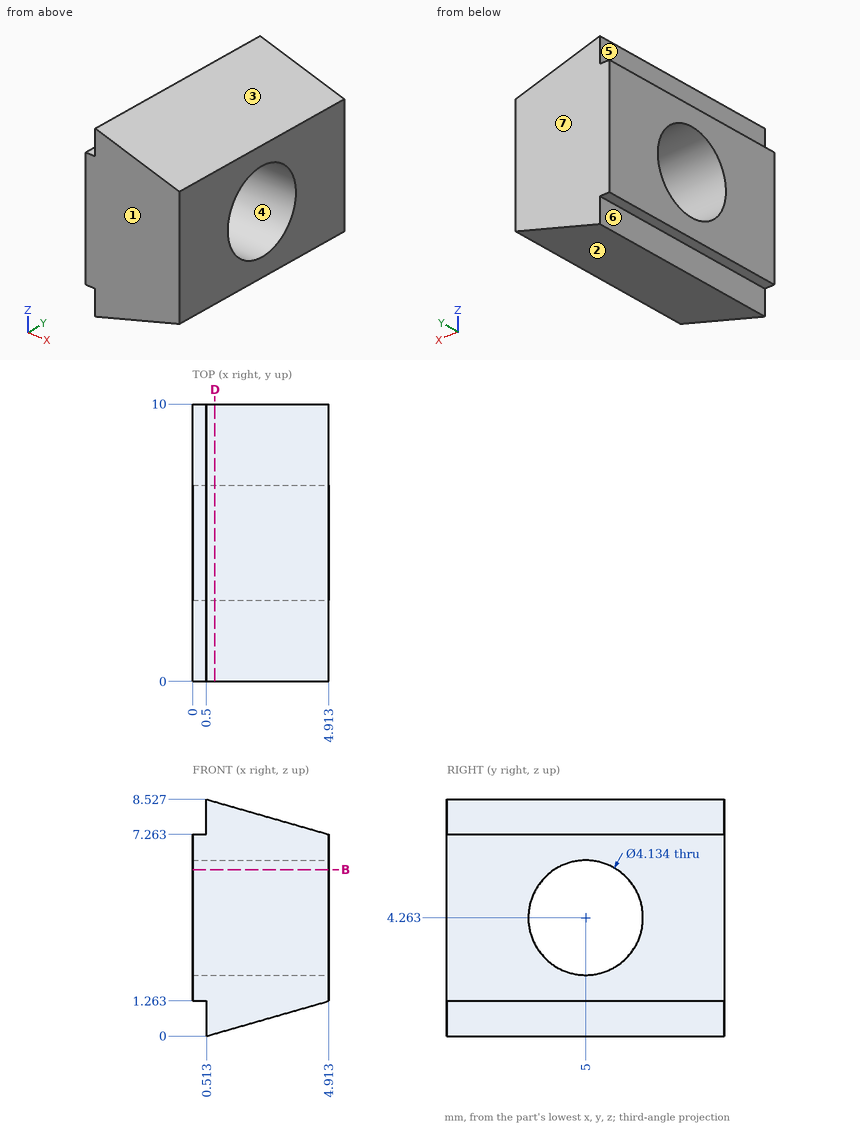
Part print with two shaded views. Sizes in mm from the minimum x, y, z corner. A direction names the side the tool comes from. Give positions to 0.01 mm unless a question says otherwise; leave off trailing zeros. Order: outer loops, then holes, each group sorted by start corner. A loop starts at its lowest first (then second) coordinate and runs counter-clockwise, first axis right, second up. Notation, with made-up numbers: (3, 84) - (19, 84) arc R23 cw to (19, 97) - close; hole circle Ø2 at (87.5, -27). An arc over 180 degrees is marked (long way). Write each question's results on one line, items separated by ' | '.
1. Saw through at D-D on x = 0.8. List the corners of the cut face in (y, z) (1 decimal), and give its area (3 significant figures).
Calculated:
outline: (0, 0.1) - (10, 0.1) - (10, 8.4) - (0, 8.4) - close; hole circle Ø4.1 at (5, 4.3) | area: 70.2 mm2
2. Pull direction Z, two halves, no side cores. Call the marked faces 1, 2, 3 and 4: released by +Z, released by -Z, zero draft, split by the parting line, or undercut.
Calculated:
face 1: zero draft | face 2: released by -Z | face 3: released by +Z | face 4: undercut
3. 3-axis set-ups, long thin cutter, end or side, ignore diameter. For the marked faces 5, 6 and 7: which of +Z, -Z, +X, -X, +Y, -Y reach the whole face in a straight line?
Calculated:
face 5: +Z, -X, +Y, -Y | face 6: -Z, -X, +Y, -Y | face 7: +Z, -Z, +X, -X, +Y
4. Pin check, flat tips, straight feed: pin 1 (1 mm diameter, centred on y = 4, z = 0.5, fed in from -X); pin 2 (1 mm diameter, centred on x = 4, z = 4, fed in from -Y). Stop position of each tip, or through.
Calculated:
pin 1: stops at x = 0.5 | pin 2: stops at y = 0
5. Probe L1, parallel to Y at x = 3.7, z = 3 (1 decimal); L2, parallel to Y at x = 3.6, z = 5.5 (1 decimal); L3, parallel to Z at x = 2.5, y = 5. List the from-to ranges inside material, lowest first. Write a range as from..to.
Calculated:
L1: y = 0..3.4, 6.6..10 | L2: y = 0..3.3, 6.7..10 | L3: z = 0.57..2.2, 6.33..7.96
6. Saw through at B-B on z = 6. List the corners of the cut face in (x, y).
Calculated:
outline: (0, 0) - (4.91, 0) - (4.91, 3.88) - (0, 3.88) - close; (0, 6.12) - (4.91, 6.12) - (4.91, 10) - (0, 10) - close
